```python
from build123d import *

# Parameters (mm, degrees)
ESBO_O1_R                  = 1
RESSALTO_EXTRUS_O1_DEPTH   = 5
CORTE_EXTRUS_O1_DEPTH      = 5
CORTE_EXTRUS_O1_DEPTH_BACK = 5
ESBO_O3_R                  = 3
CORTE_EXTRUS_O2_DEPTH      = 1


with BuildPart() as part:
    # Esboço1 → Ressalto-extrusão1 (new body)
    with BuildSketch(Plane.XY):
        with BuildLine():
            Line((4.3972248, -0.95625), (0.244290267, -20.053125))
            ThreePointArc((0.244290267, -20.053125), (0, -20.25), (-0.244290267, -20.053125))
            Line((-0.244290267, -20.053125), (-4.3972248, -0.95625))
            ThreePointArc((-4.3972248, -0.95625), (0, 4.5), (4.3972248, -0.95625))
        make_face()
        Circle(ESBO_O1_R, mode=Mode.SUBTRACT)
    extrude(amount=RESSALTO_EXTRUS_O1_DEPTH)

    # Esboço2 → Corte-extrusão1 (cut, two sides: drawn at the far end of the back side and taken through both)
    with BuildSketch(Plane(origin=(0, 0, 0), x_dir=(0, 0, -1), z_dir=(1, 0, 0)).offset(-CORTE_EXTRUS_O1_DEPTH_BACK)):
        Polygon((0, 4.5), (0, -20.25), (-4.5, -20.25), (-1, 4.5), align=None)
    extrude(amount=CORTE_EXTRUS_O1_DEPTH + CORTE_EXTRUS_O1_DEPTH_BACK, mode=Mode.SUBTRACT)

    # Esboço3 → Corte-extrusão2 (cut)
    with BuildSketch(Plane.XY.offset(5)):
        Circle(ESBO_O3_R)
    extrude(amount=-CORTE_EXTRUS_O2_DEPTH, mode=Mode.SUBTRACT)


solid = part.part
```
For this review, take the finished solid that the model builds, in its own axes (mm). A direction names the side the tool comes from. Coordinates: 2 decimals unless noted, no trailing zeros. Loops run counter-clockwise (first coordinate to the right, second up) from the corner with the lowest first, then second, coordinate; pieces in that order, holes last.
1. Mouldability with a two-part tool opening along Y and no side actions: class faces 1 (the flat face through (2.81, -8.25, 3.72)), 2 (the flat face through (0, -5, 5)), 3 (the cylindrical face through (-3, 0.1, 4.5)) as +Y half, -Y half, draft (parallel to the pull), parting line (faces both ways), or undercut.
2. Add section D-D, the plane y = -14.75. Give the boundary of the cut face in (x, z), then the cut area to 3 significant figures.
3. Insertion check: P1, Ø4, axis at x = 0, y = -15, coming from the -Z side; P2, Ø1.5, axis at y = -10.5, z = 1.5, coming from the -X side; P3, Ø1, axis at x = 1.5, y = -6.5, coming from the -Z side; P4, Ø2.5, axis at x = 0, y = 0, coming from the -Z side. Each pin has a flat end and moves straight along its axis. Give the tip position at first contact, or say it passes through.
4. Add section C-C, the plane z = 2.9. Give the boundary of the cut face in (x, y), then the cut area to 3 significant figures.
5. For faces 4 (the flat face through (-1, 1, 4)), 5 (the flat face through (-2.753, -8.516, 3.722)), list the 3-axis set-ups (+Z, -Z, +X, -X, +Y, -Y) from which the entire face can be reached by the end or side of a thin tool; tool diameter is ignored.
6. Add section B-B, the plane x = 0. Give the boundary of the cut face in (y, z), then the cut area to 3 significant figures.
7. For line 1 (X direction, y = 0, z = 2.6); line 2 (Y direction, x = 0, z = 4.7); line 3 (X direction, y = -3.5, z = 2.7), list the stretches that pass through material, from the lowest coordinate up.
8. Add section A-A, the plane y = 0. Give the boundary of the cut face in (x, z).
Result:
1. face 1: -Y half
1. face 2: draft
1. face 3: undercut
2. outline: (-1.4, 3.72) - (1.4, 3.72) - (1.4, 5) - (-1.4, 5) - close
2. area: 3.57 mm2
3. P1: stops at z = 3.47
3. P2: passes through
3. P3: stops at z = 2.48
3. P4: stops at z = 1.46
4. outline: (-4.4, -0.96) - (-2.66, -8.94) - (2.66, -8.94) - (4.4, -0.96) arc R4.5 ccw (long way) to start; hole circle Ø2 at (0, 0)
4. area: 93.5 mm2
5. face 4: +Z
5. face 5: +Z, -Z, -X, -Y
6. outline: (-20.25, 4.5) - (-1, 1.78) - (-1, 4) - (-3, 4) - (-3, 5) - (-20.25, 5) - close; (1, 1.49) - (4.5, 1) - (4.5, 5) - (3, 5) - (3, 4) - (1, 4) - close
6. area: 45.0 mm2
7. line 1: x = -4.5 to -1, 1 to 4.5
7. line 2: y = -20.25 to -3, 3 to 4.5
7. line 3: x = -3.84 to 3.84
8. outline: (-4.5, 1.64) - (-1, 1.64) - (-1, 4) - (-3, 4) - (-3, 5) - (-4.5, 5) - close; (1, 1.64) - (4.5, 1.64) - (4.5, 5) - (3, 5) - (3, 4) - (1, 4) - close
